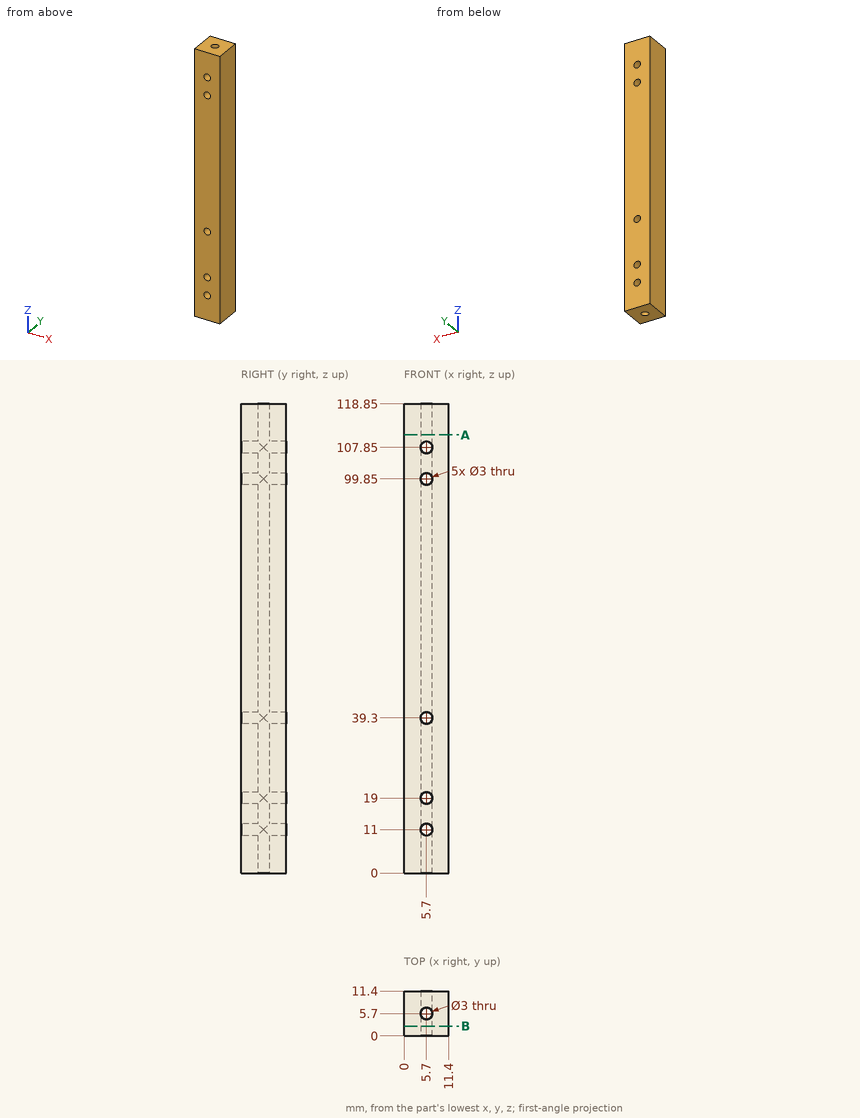
The drawing under review shows one solid part. Ordinate dimensions are in mm from its lowest x, y, z. Round coordinates to 2 decimals unless told otherwise and drop trailing zeros. Order: outer loops, then holes, each group sorted by start corner. A loop starts at its lowest first (then second) coordinate and runs counter-clockwise, first axis right, second up. Notation, with made-up numbers: (-7, 56) - (38, 56) arc R15 cw to (38, 64) - close; hole circle Ø1 at (12.5, -5.5). An arc over 180 degrees is marked (long way). Return JSON: item names as keys, results as strings.
Q1. Wall thickness on L1, parallel to X at y = 8.1, z = 11; L2, parallel to Z at x = 4.75, y = 11: over which ranges is each line inside the solid? List them lowest first. Write a range as [from, to].
Computed values:
{"L1": "x = [0, 4.2], [7.2, 11.4]", "L2": "z = [0, 9.84], [12.16, 17.84], [20.16, 38.14], [40.46, 98.69], [101.01, 106.69], [109.01, 118.85]"}
Q2. For pin 1 Ø2.5 at (x, z) = (5.7, 39.3) entering from -Y, flat-tipped, find the tip position at first contact; note if it passes through.
Computed values:
{"pin 1": "passes through"}
Q3. Consider section A-A on z = 111. Write out the cut boundary in (x, y), plus the area to 3 significant figures.
Computed values:
{"outline": "(0, 0) - (11.4, 0) - (11.4, 11.4) - (0, 11.4) - close; hole circle Ø3 at (5.7, 5.7)", "area": "123 mm2"}
Q4. Consider section B-B on y = 2.5. Write out the cut boundary in (x, z), plus the area to 3 significant figures.
Computed values:
{"outline": "(0, 0) - (11.4, 0) - (11.4, 118.85) - (0, 118.85) - close; hole circle Ø3 at (5.7, 11); hole circle Ø3 at (5.7, 19); hole circle Ø3 at (5.7, 39.3); hole circle Ø3 at (5.7, 99.85); hole circle Ø3 at (5.7, 107.85)", "area": "1,320 mm2"}
